from build123d import *

# Parameters (mm, degrees)
SKETCH010_R      = 2.9
EXTRUDE010_DEPTH = 20
SKETCH009_W      = 20
SKETCH009_H      = 7.87
EXTRUDE009_DEPTH = 90


with BuildPart() as tornillos003:
    # Sketch010 (on Face4 of Extrude009) → Extrude010 (new body)
    with BuildSketch(Plane.XY.offset(19.952513)):
        with Locations((10, -80)):
            Circle(SKETCH010_R)
        with Locations((10, -45.010692)):
            Circle(SKETCH010_R)
        with Locations((10, -10.021384)):
            Circle(SKETCH010_R)
    extrude(amount=EXTRUDE010_DEPTH)


with BuildPart() as tornillos003_1:
    # Extrude010 placement: moved
    add(tornillos003.part.moved(Location((0, 0, -15))))


with BuildPart() as cut:
    # Sketch009 → Extrude009 (new body)
    with BuildSketch(Plane.XZ):
        with Locations((10.003101, 16.017513)):
            Rectangle(SKETCH009_W, SKETCH009_H)
    extrude(amount=EXTRUDE009_DEPTH)

    # Cut: cut Tornillos003
    add(tornillos003_1.part, mode=Mode.SUBTRACT)


solid = cut.part
Geometry: final body of the model. Coordinates: model frame, mm. Round coordinates to 2 decimals unless told otherwise and drop trailing zeros. Write each loop counter-clockwise with the first axis right and the second up, starting at its lowest first coordinate (ties: lowest second). Pieces come first, ordered by that corner, then holes. Notation, with made-up numbers: M -34,68 L 18,68 A5 ccw 18,76 Z; hole C -8.75,15 d4. An arc over 180 degrees is marked long. Write item = value, one per line.
Item 1: Pull-direction query (Y, two-part tool) for faces 1 (the face through (7.699, -81.765, 15.962)), 2 (the face through (10, -90, 16)), 3 (the face through (5, -44, 12.083)); classes: pulls with the +Y half, pulls with the -Y half, needs draft (parallel to the pull), parting line crosses it, or undercut.
Findings:
face_1 = undercut
face_2 = pulls with the -Y half
face_3 = needs draft
Item 2: Section query C-C on z = 17.25. Return loops of the section in (x, y).
Findings:
outline = M 0,-90 L 20,-90 L 20,0 L 0,0 Z; hole C 10,-80 d5.8; hole C 10,-45.01 d5.8; hole C 10,-10.02 d5.8
Item 3: Section query B-B on x = 10. Return loops of the section in (y, z).
Findings:
outline = M -90,12.08 L -82.9,12.08 L -82.9,19.95 L -90,19.95 Z; M -77.1,12.08 L -47.91,12.08 L -47.91,19.95 L -77.1,19.95 Z; M -42.11,12.08 L -12.92,12.08 L -12.92,19.95 L -42.11,19.95 Z; M -7.12,12.08 L 0,12.08 L 0,19.95 L -7.12,19.95 Z
Item 4: Section query A-A on y = -80. Return loops of the section in (x, z).
Findings:
outline = M 0,12.08 L 7.1,12.08 L 7.1,19.95 L 0,19.95 Z; M 12.9,12.08 L 20,12.08 L 20,19.95 L 12.9,19.95 Z
Item 5: Section query D-D on y = -8.5. Return loops of the section in (x, z).
Findings:
outline = M 0,12.08 L 7.53,12.08 L 7.53,19.95 L 0,19.95 Z; M 12.47,12.08 L 20,12.08 L 20,19.95 L 12.47,19.95 Z
Item 6: Pin query (flat end, axial travel): P1, Ø4.5, axis at x = 10, y = -45.01, coming from the +Z side (3 decimals); P2, Ø1, axis at x = 15, z = 14, coming from the +Y side. Return the tip coordinate at first contact, or that it passes through.
Findings:
P1 = through
P2 = 0
Item 7: Material intervals for line 1 along Y through (x, z) = (10, 17.75); line 2 along X through (y, z) = (-80, 16); line 3 along Y through (x, z) = (12, 15.5), sorted ascending. Write a range as [from, to].
Findings:
line_1 = [-90, -82.9], [-77.1, -47.91], [-42.11, -12.92], [-7.12, 0]
line_2 = [0, 7.1], [12.9, 20]
line_3 = [-90, -82.1], [-77.9, -47.11], [-42.91, -12.12], [-7.92, 0]
